from build123d import *

# Parameters (mm, degrees)
SALIENTE_EXTRUIR2_DEPTH = 15
CORTAR_EXTRUIR5_START   = -126
CORTAR_EXTRUIR5_DEPTH   = 126
CORTAR_EXTRUIR6_DEPTH   = 13


# Read off the part's stored shape, not the designer's step: Cortar-Extruir5
with BuildPart() as part:
    # Croquis1 → Saliente-Extruir2 (new body)
    with BuildSketch(Plane(origin=(0, 0, 0), x_dir=(1, 0, 0), z_dir=(0, 1, 0))):
        with BuildLine():
            Line((0, 0), (2, 0))
            Line((2, 0), (2, -11))
            Line((2, -11), (128, -11))
            Line((128, -11), (128, 0))
            Line((128, 0), (130, 0))
            Line((130, 0), (130, 187))
            ThreePointArc((130, 187), (128.828427125, 189.828427125), (126, 191))
            Line((126, 191), (4, 191))
            ThreePointArc((4, 191), (1.171572875, 189.828427125), (0, 187))
            Line((0, 187), (0, 0))
        make_face()
    extrude(amount=SALIENTE_EXTRUIR2_DEPTH)

    # Cortar-Extruir5 outline → Cortar-Extruir5 (cut)
    with BuildSketch(Plane(origin=(128, 0, 0), x_dir=(0, 0, -1), z_dir=(1, 0, 0)).offset(CORTAR_EXTRUIR5_START)):
        with BuildLine():
            Line((-11, 0), (-3.5, 0))
            ThreePointArc((-3.5, 0), (-8.803300859, 2.196699141), (-11, 7.5))
            Line((-11, 7.5), (-11, 0))
        make_face()
        with BuildLine():
            Line((-11, 15), (-11, 7.5))
            ThreePointArc((-11, 7.5), (-8.803300859, 12.803300859), (-3.5, 15))
            Line((-3.5, 15), (-11, 15))
        make_face()
    extrude(amount=CORTAR_EXTRUIR5_DEPTH, mode=Mode.SUBTRACT)

    # Croquis3 → Cortar-Extruir6 (cut)
    with BuildSketch(Plane(origin=(0, 15, 0), x_dir=(1, 0, 0), z_dir=(0, 1, 0))):
        with BuildLine():
            Line((2, 80.037921952), (2, 185))
            ThreePointArc((2, 185), (3.171572875, 187.828427125), (6, 189))
            Line((6, 189), (124, 189))
            ThreePointArc((124, 189), (126.828427125, 187.828427125), (128, 185))
            Line((128, 185), (128, 95.850744251))
            Line((128, 95.850744251), (128, 2))
            Line((128, 2), (126, 2))
            Line((126, 2), (126, -1.75))
            Line((126, -1.75), (57.409845297, -1.5))
            Line((57.409845297, -1.5), (4, -1.75))
            Line((4, -1.75), (4, 2))
            Line((4, 2), (2, 2))
            Line((2, 2), (2, 80.037921952))
        make_face()
    extrude(amount=-CORTAR_EXTRUIR6_DEPTH, mode=Mode.SUBTRACT)


solid = part.part
The listing builds one solid part. Answer for the finished solid, in the listing's coordinates (mm). A direction names the side the tool comes from. Coordinates: 2 decimals unless noted, no trailing zeros. Order: outer loops, then holes, each group sorted by start corner. A loop starts at its lowest first (then second) coordinate and runs counter-clockwise, first axis right, second up. Notation, with made-up numbers: (-18.75, 58.25) -> (7.25, 58.25) arc R9 cw to (7.25, 74.25) -> close; hole circle Ø9 at (32, 21). An arc over 180 degrees is marked (long way). Answer in a Markdown table with one row per item. Add a question column.
Item 1: Find section D-D (x = 9.5). Write down the section's boundary in (y, z).
Item 2: Find the intervals of material crossed by L1, parallel to X at y = 6.75, z = -71; L2, parallel to Z at x = 66.5, y = 7.75; L3, parallel to Y at x = 89.5, z = -161.5, in increasing order. Write a range as from..to.
Item 3: Find section A-A (z = -161). Write down the section's boundary in (x, y), then the cut area to 3 significant figures.
Item 4: Which of the six approach directions +Z, -Z, +X, -X, +Y, -Y give full straight-line access (tool end or side, diameter ignored) to faces 4 (the face through (2, 7, 4)), 5 (the face through (128, 9, -95)), 6 (the face through (128, 7, 4)), 7 (the face through (128.859, 7.395, -189.797)), 8 (the face through (64, 0, -95))?
Item 5: Find section C-C (x = 45.5). Write down the section's boundary in (y, z).
Item 6: Each of these flat-tipped pins is pushed along its axis until it touches: P1, Ø2, axis at x = 128.5, y = 9.5, coming from the +Z side; P2, Ø2, axis at x = 50.5, z = -90, coming from the +Y side; P3, Ø1, axis at x = 127.5, y = 6, coming from the -Z side. Where does it stop, or does it pass through?
Item 7: Determine the mould class of faces 1 (the face through (1.203, 7.395, -189.859)), 2 (the face through (126.797, 8.591, -187.859)), 3 (the face through (130, 7, -92)) for opening direction X: +X half, -X half, draft (parallel to the pull), parting line (faces both ways), or undercut.
Item 8: Find section B-B (y = 12.25). Write down the section's boundary in (x, z), then the cut area to 3 significant figures.
Result set:
| question | item | result |
|---|---|---|
| 1 | outline | (0, -191) -> (15, -191) -> (15, -189) -> (2, -189) -> (2, 1.72) -> (15, 1.72) -> (15, 3.5) arc R7.5 ccw to (0, 3.5) -> close |
| 2 | L1 | x = 0..2, 128..130 |
| 2 | L2 | z = -191..-189, 1.53..11 |
| 2 | L3 | y = 0..2 |
| 3 | outline | (0, 0) -> (130, 0) -> (130, 15) -> (128, 15) -> (128, 2) -> (2, 2) -> (2, 15) -> (0, 15) -> close |
| 3 | area | 312 mm² |
| 4 | face 4 | +Z, -X, +Y, -Y |
| 4 | face 5 | +Y |
| 4 | face 6 | +Z, +X, +Y, -Y |
| 4 | face 7 | -Z, +X, +Y, -Y |
| 4 | face 8 | +Z, -Z, +X, -X, -Y |
| 5 | outline | (0, -191) -> (15, -191) -> (15, -189) -> (2, -189) -> (2, 1.56) -> (15, 1.56) -> (15, 3.5) arc R7.5 ccw to (0, 3.5) -> close |
| 6 | P1 | stops at z = 10.91 |
| 6 | P2 | stops at y = 2 |
| 6 | P3 | stops at z = -190.87 |
| 7 | face 1 | -X half |
| 7 | face 2 | undercut |
| 7 | face 3 | +X half |
| 8 | outline | (0, -187) arc R4 ccw to (4, -191) -> (126, -191) arc R4 ccw to (130, -187) -> (130, 0) -> (128, 0) -> (128, 9.3) -> (2, 9.3) -> (2, 0) -> (0, 0) -> close; hole (2, -185) arc R4 ccw to (6, -189) -> (124, -189) arc R4 ccw to (128, -185) -> (128, -2) -> (126, -2) -> (126, 1.75) -> (57.41, 1.5) -> (4, 1.75) -> (4, -2) -> (2, -2) -> close |
| 8 | area | 2,000 mm² |
